```python
from build123d import *

# Parameters (mm, degrees)
F7_R      = 960.2431856589
F8_DEPTH  = 635.5163904251
F12_R     = 870.2287794889
F13_DEPTH = 25
F14_R     = 892.9375722879
F15_DEPTH = 25
F19_REACH = 935.9843056137
F20_DEPTH = 216.5073510461
F23_DEPTH = 25


with BuildPart() as f5:
    # F3 (on Top) → F5 section 0
    with BuildSketch(Plane.XY):
        Polygon((-375, -216.5063509461), (375, -216.5063509461), (0, 433.0127018922), align=None)
    # F4 (on line) → F5 section 1
    with BuildSketch(Plane.XY.offset(1650)):
        Polygon((-150, -86.6025403784), (150, -86.6025403784), (0, 173.2050807569), align=None)
    loft()

    # F7 (on face) → F8 (cut, through all)
    with BuildSketch(Plane(origin=(0, -203.2096543416, 15.9986111776), x_dir=(1, 0, 0), z_dir=(0, -0.9969151597, 0.078486714))):
        with Locations((0, 812.9688501358)):
            Circle(F7_R)
    extrude(amount=-F8_DEPTH, mode=Mode.SUBTRACT)

    # F12 (on face) → F13 (cut)
    with BuildSketch(Plane(origin=(0, 0, 0), x_dir=(0.8660254038, -0.5, 0), z_dir=(-0.5, -0.8660254038, 0))):
        with Locations((304.0688931942, 817.2121047974)):
            Circle(F12_R)
    extrude(amount=-F13_DEPTH, mode=Mode.SUBTRACT)

    # F14 (on face) → F15 (cut)
    with BuildSketch(Plane(origin=(0, 0, 0), x_dir=(-0.8660254038, -0.5, 0), z_dir=(-0.5, 0.8660254038, 0))):
        with Locations((291.6465699673, 811.1194968224)):
            Circle(F14_R)
    extrude(amount=F15_DEPTH, mode=Mode.SUBTRACT)

    f19_end = Plane(origin=(0, -155.5781982198, 697.4454188962), x_dir=(0, 0.078486714, 0.9969151597), z_dir=(0, 0.9969151597, -0.078486714))
    # F17 (on Front) → F19 (cut, up to a plane its end follows)
    with BuildSketch(Plane.XZ):
        Polygon((-181.3636363636, 1420), (181.3636363636, 1420), (179.7272727273, 1432), (-179.7272727273, 1432), align=None)
        Polygon((151.6363636364, 1638), (150, 1650), (-150, 1650), (-151.6363636364, 1638), align=None)
        Polygon((308.4545454545, 488), (306.8181818182, 500), (-306.8181818182, 500), (-308.4545454545, 488), align=None)
        Polygon((-365.4545454545, 70), (365.4545454545, 70), (363.8181818182, 82), (-363.8181818182, 82), align=None)
    f19_long = extrude(amount=F19_REACH, mode=Mode.PRIVATE)
    add(split(f19_long, bisect_by=f19_end, keep=Keep.TOP, mode=Mode.PRIVATE), mode=Mode.SUBTRACT)

    # F16 (on Front) → F20 (cut, through all)
    with BuildSketch(Plane.XZ):
        Polygon((-267.2563485856, 50), (-274.0745304038, 0), (274.0745304038, 0), (267.2563485856, 50), align=None)
        Polygon((-205.8927122219, 500), (205.8927122219, 500), (83.1654394947, 1400), (-83.1654394947, 1400), align=None)
    extrude(amount=F20_DEPTH, mode=Mode.SUBTRACT)

    # F22 (on face) → F23 (join)
    with BuildSketch(Plane(origin=(0, 0, 0), x_dir=(-0.8660254038, -0.5, 0), z_dir=(-0.5, 0.8660254038, 0))):
        Polygon((160.2172859615, 1639.4481457139), (151.0203254662, 1638), (153.2218541075, 1624.0184153092), (162.4188146029, 1625.4665610231), align=None)
    extrude(amount=F23_DEPTH)


solid = f5.part
```
Part model, mm, in its own coordinate system. Coordinates: 2 decimals unless noted, no trailing zeros. Put each result on its own line as item: value. Start each with the question number.
(1) Pin check, flat tips, straight feed: pin 1 Ø3 at (x, y) = (26.5, -78) entering from +Z; pin 2 Ø5 at (x, y) = (24.5, -172.5) entering from +Z; pin 3 Ø3 at (x, y) = (137, -168) entering from +Z. Stop position of each tip, or through.
(2) Probe line 1 along X through (y, z) = (-121.5, 1080.5); line 2 along X through (y, z) = (-180, 417.5); line 3 along Y through (x, z) = (-286, 453.5). List the from-to ranges inside material, lowest first. Write a range as [from, to].
(3) Mould opens along X. For faces 1 (the face through (144.815, -135.501, 947.9)), 2 (the face through (252.324, -145.679, 828.85)), 3 (the face through (146.95, -128.72, 962.15)), 4 (the face through (-253.28, -146.23, 767.74)) say: pulls with the +X half, pulls with the -X half, needs draft (parallel to the pull), parting line crosses it, or undercut.
Determined:
1. pin 1: stops at z = 1638
1. pin 2: stops at z = 500
1. pin 3: stops at z = 488
2. line 1: x = [-210.44, -126.73], [126.73, 210.44]
2. line 2: x = [-311.77, 311.77]
2. line 3: y = [-180.8, -168.77]
3. face 1: undercut
3. face 2: pulls with the +X half
3. face 3: needs draft
3. face 4: pulls with the -X half
